```python
from build123d import *

# Parameters (mm, degrees)
F0_W     = 191.3
F0_H     = 69.5
F0_R     = 1.6
F0_R_2   = 2.55
F0_R_3   = 6.1
F0_R_4   = 1.3
F0_W_2   = 33
F0_H_2   = 44
F1_DEPTH = 1.5


with BuildPart() as f1:
    # F0 (on Top) → F1 (new body)
    with BuildSketch(Plane.XY):
        with Locations((90, 30)):
            Rectangle(F0_W, F0_H)
        with Locations((9, 5)):
            Circle(F0_R, mode=Mode.SUBTRACT)
        with Locations((10, 28)):
            Circle(F0_R_2, mode=Mode.SUBTRACT)
        with Locations((83, 28)):
            Circle(F0_R_3, mode=Mode.SUBTRACT)
        with Locations((107.5, 10.2)):
            Circle(F0_R_4, mode=Mode.SUBTRACT)
        with Locations((172.5, 10.2)):
            Circle(F0_R_4, mode=Mode.SUBTRACT)
        Polygon((175.8, 13.2), (104.2, 13.2), (104.2, 20.3), (100.1, 20.3), (100.1, 40.3), (104.2, 40.3), (175.8, 40.3), align=None, mode=Mode.SUBTRACT)
        with Locations((35.5, 33)):
            Rectangle(F0_W_2, F0_H_2, mode=Mode.SUBTRACT)
        with Locations((9, 55)):
            Circle(F0_R, mode=Mode.SUBTRACT)
        with Locations((83, 48)):
            Circle(F0_R_2, mode=Mode.SUBTRACT)
        with Locations((107.5, 43.3)):
            Circle(F0_R_4, mode=Mode.SUBTRACT)
        with Locations((172.5, 43.3)):
            Circle(F0_R_4, mode=Mode.SUBTRACT)
        with Locations((120, 52)):
            Circle(F0_R_2, mode=Mode.SUBTRACT)
        with Locations((140, 52)):
            Circle(F0_R_2, mode=Mode.SUBTRACT)
        with Locations((160, 52)):
            Circle(F0_R_2, mode=Mode.SUBTRACT)
    extrude(amount=F1_DEPTH)


solid = f1.part
```
The listing builds one solid part. Answer for the finished solid, in the listing's coordinates (mm). Give positions to 0.01 mm unless a question says otherwise; leave off trailing zeros. Order: outer loops, then holes, each group sorted by start corner. A loop starts at its lowest first (then second) coordinate and runs counter-clockwise, first axis right, second up. Notation, with made-up numbers: (64.25, 64.5) - (102.25, 64.5) arc R28 cw to (102.25, 84.5) - close; hole circle Ø7 at (18.5, 17.25). An arc over 180 degrees is marked (long way). Answer in a Markdown table with one row per item. Add a question column.
Q1. The part is cut by section B-B (x = 120). Determine the outline of the cut face in (y, z), then the cut area to 4 significant figures.
Q2. Given P1, Ø3, axis at x = 129, y = 48, coming from the -Z side, flat-ended and moving along its own axis, determine where the tip first touches the part or whether it passes through.
Q3. The part is cut by section C-C (z = 0.4). Give the number of separate pieces and of enclosed holes in the cut face, then the cut area to 3 significant figures.
Q4. Find the intervals of material crossed by line 1 along Y through (x, z) = (120, 1.15); line 2 along Y through (x, z) = (107.5, 0.95); line 3 along X through (y, z) = (16.5, 0.5), in increasing order. Write a range as [from, to].
Q5. The part is cut by section D-D (x = 29.5). Determine the outline of the cut face in (y, z).
Q6. For a pull along Y with two mould halves and no side action, classify faces 1 (the flat face through (89, 30, 0)), 2 (the cylindrical face through (86.279, 33.144, 0.74)) as released by +Y, released by -Y, zero draft, split by the parting line, or undercut.
Q7. The part is cut by section A-A (y = 28). Determine the outline of the cut face in (x, z).
Determined:
| question | item | result |
|---|---|---|
| 1 | outline | (-4.75, 0) - (13.2, 0) - (13.2, 1.5) - (-4.75, 1.5) - close; (40.3, 0) - (49.45, 0) - (49.45, 1.5) - (40.3, 1.5) - close; (54.55, 0) - (64.75, 0) - (64.75, 1.5) - (54.55, 1.5) - close |
| 1 | area | 55.95 mm² |
| 2 | P1 | stops at z = 0 |
| 3 | separate pieces | 1 |
| 3 | enclosed holes | 14 |
| 3 | area | 9,560 mm² |
| 4 | line 1 | y = [-4.75, 13.2], [40.3, 49.45], [54.55, 64.75] |
| 4 | line 2 | y = [-4.75, 8.9], [11.5, 13.2], [40.3, 42], [44.6, 64.75] |
| 4 | line 3 | x = [-5.65, 19], [52, 104.2], [175.8, 185.65] |
| 5 | outline | (-4.75, 0) - (11, 0) - (11, 1.5) - (-4.75, 1.5) - close; (55, 0) - (64.75, 0) - (64.75, 1.5) - (55, 1.5) - close |
| 6 | face 1 | zero draft |
| 6 | face 2 | undercut |
| 7 | outline | (-5.65, 0) - (7.45, 0) - (7.45, 1.5) - (-5.65, 1.5) - close; (12.55, 0) - (19, 0) - (19, 1.5) - (12.55, 1.5) - close; (52, 0) - (76.9, 0) - (76.9, 1.5) - (52, 1.5) - close; (89.1, 0) - (100.1, 0) - (100.1, 1.5) - (89.1, 1.5) - close; (175.8, 0) - (185.65, 0) - (185.65, 1.5) - (175.8, 1.5) - close |
